```python
from build123d import *

# Parameters (mm, degrees)
SKETCH_1_R      = 1.5
EXTRUDE_1_DEPTH = 4


with BuildPart() as part:
    # 草图1 → 凸台-拉伸1 (new body)
    with BuildSketch(Plane.XY):
        with BuildLine():
            Line((46.801771952, 35.924840183), (49.578148254, 38.05597477))
            ThreePointArc((49.578148254, 38.05597477), (-61.863840118, -8.894677392), (58.29149197, -22.546661925))
            Line((58.29149197, -22.546661925), (55.027168419, -21.284048857))
            ThreePointArc((55.027168419, -21.284048857), (50.484575742, -23.055533222), (52.120542762, -27.648671255))
            ThreePointArc((52.120542762, -27.648671255), (44.589224887, -38.636783303), (34.784774262, -47.65521461))
            ThreePointArc((34.784774262, -47.65521461), (30.005565369, -46.689571072), (28.898590503, -51.438035217))
            ThreePointArc((28.898590503, -51.438035217), (16.622220854, -56.610085443), (3.498460053, -58.896186441))
            ThreePointArc((3.498460053, -58.896186441), (0, -55.5), (-3.498460053, -58.896186441))
            ThreePointArc((-3.498460053, -58.896186441), (-16.622220854, -56.610085443), (-28.898590503, -51.438035217))
            ThreePointArc((-28.898590503, -51.438035217), (-30.005565369, -46.689571072), (-34.784774262, -47.65521461))
            ThreePointArc((-34.784774262, -47.65521461), (-44.589224887, -38.636783303), (-52.120542762, -27.648671255))
            ThreePointArc((-52.120542762, -27.648671255), (-50.484575742, -23.055533222), (-55.027168419, -21.284048857))
            ThreePointArc((-55.027168419, -21.284048857), (-58.399465071, -8.396575458), (-58.794590961, 4.918950474))
            ThreePointArc((-58.794590961, 4.918950474), (-54.935090024, 7.898473524), (-57.798825407, 11.844652023))
            ThreePointArc((-57.798825407, 11.844652023), (-53.668287726, 24.509485767), (-46.801771952, 35.924840183))
            ThreePointArc((-46.801771952, 35.924840183), (-41.944101377, 36.344770734), (-42.219763715, 41.212759575))
            ThreePointArc((-42.219763715, 41.212759575), (-31.89780823, 49.633958437), (-19.949721034, 55.524846967))
            ThreePointArc((-19.949721034, 55.524846967), (-15.636156905, 53.251860036), (-13.236225354, 57.496107158))
            ThreePointArc((-13.236225354, 57.496107158), (0, 59), (13.236225354, 57.496107158))
            ThreePointArc((13.236225354, 57.496107158), (15.636156905, 53.251860036), (19.949721034, 55.524846967))
            ThreePointArc((19.949721034, 55.524846967), (31.89780823, 49.633958437), (42.219763715, 41.212759575))
            ThreePointArc((42.219763715, 41.212759575), (41.944101377, 36.344770734), (46.801771952, 35.924840183))
        make_face()
        with Locations((0, -59)):
            Circle(SKETCH_1_R, mode=Mode.SUBTRACT)
        with Locations((-31.89780823, -49.633958437)):
            Circle(SKETCH_1_R, mode=Mode.SUBTRACT)
        with Locations((-53.668287726, -24.509485767)):
            Circle(SKETCH_1_R, mode=Mode.SUBTRACT)
        with Locations((-58.399465071, 8.396575458)):
            Circle(SKETCH_1_R, mode=Mode.SUBTRACT)
        with Locations((-44.589224887, 38.636783303)):
            Circle(SKETCH_1_R, mode=Mode.SUBTRACT)
        with Locations((-16.622220854, 56.610085443)):
            Circle(SKETCH_1_R, mode=Mode.SUBTRACT)
        with Locations((16.622220854, 56.610085443)):
            Circle(SKETCH_1_R, mode=Mode.SUBTRACT)
        with Locations((44.589224887, 38.636783303)):
            Circle(SKETCH_1_R, mode=Mode.SUBTRACT)
        with Locations((53.668287726, -24.509485767)):
            Circle(SKETCH_1_R, mode=Mode.SUBTRACT)
        with Locations((31.89780823, -49.633958437)):
            Circle(SKETCH_1_R, mode=Mode.SUBTRACT)
    extrude(amount=EXTRUDE_1_DEPTH)


solid = part.part
```
Source: CAD feature listing. Evaluate the final solid. Frame: model axes, mm. A direction names the side the tool comes from. Round coordinates to 2 decimals unless told otherwise and drop trailing zeros. Loops run counter-clockwise (first coordinate to the right, second up) from the corner with the lowest first, then second, coordinate; pieces in that order, holes last.
(1) Access query for faces 1 (the cylindrical face through (-44.467, -38.778, 1.972)), 2 (the flat face through (56.682, -21.924, 1.972)). Directions: +Z, -Z, +X, -X, +Y, -Y. A direction counts if a zero-diameter tool reaches every point of the face in a straight line with its end or side. Return the directions, or none.
From the geometry:
face 1: +Z, -Z
face 2: +Z, -Z, +X, +Y
(2) Contact query for flat-ended pins moving along their axis: pin 1 Ø2.5 at (x, y) = (0, -59) entering from -Z; pin 2 Ø1.5 at (y, z) = (-20, 0.5) entering from -X; pin 3 Ø1.5 at (x, z) = (-17, 3.5) entering from -Y; pin 4 Ø2 at (y, z) = (-27.5, 3) entering from -X. Output: stop coordinate, or through.
From the geometry:
pin 1: passes through
pin 2: stops at x = -59.46
pin 3: stops at y = -60.35
pin 4: stops at x = -56.6
(3) Section query A-A (x = 0). Output: boundary loops of the cut face in (y, z).
From the geometry:
outline: (-62.5, 0) - (-60.5, 0) - (-60.5, 4) - (-62.5, 4) - close; (-57.5, 0) - (-55.5, 0) - (-55.5, 4) - (-57.5, 4) - close; (59, 0) - (62.5, 0) - (62.5, 4) - (59, 4) - close
(4) Pull-direction query (X, two-part tool) for faces 3 (the flat face through (48.2, 37, 2)), 4 (the cylindrical face through (-56.97, 8.85, 1.97)), 5 (the flat face through (-52, -23, 0)); classes: +X half, -X half, draft (parallel to the pull), parting line (faces both ways), or undercut.
From the geometry:
face 3: +X half
face 4: undercut
face 5: draft
(5) Section query D-D (z = 0.9). Give the number of separate pieces and of enclosed holes in the cut face, and give its area (3 significant figures).
From the geometry:
separate pieces: 1
enclosed holes: 10
area: 1,240 mm2
(6) Section query B-B (y = 43). Output: boundary loops of the cut face in (x, z).
From the geometry:
outline: (-45.36, 0) - (-40.4, 0) - (-40.4, 4) - (-45.36, 4) - close; (40.4, 0) - (45.36, 0) - (45.36, 4) - (40.4, 4) - close
(7) Section query C-C (x = 38.5). Output: boundary loops of the cut face in (y, z), and give its area (3 significant figures).
From the geometry:
outline: (-49.23, 0) - (-44.71, 0) - (-44.71, 4) - (-49.23, 4) - close; (44.71, 0) - (49.23, 0) - (49.23, 4) - (44.71, 4) - close
area: 36.2 mm2
(8) Material intervals for probe 1 along Y at (x, z) = (-43.5, 0.8); probe 2 along X at (y, z) = (-24, 1.65); probe 3 along Y at (x, z) = (32.5, 3.7), sorted ascending.
From the geometry:
probe 1: y = -44.88 to -39.86, 35.31 to 37.61, 39.67 to 44.88
probe 2: x = -57.71 to -55.08, -52.26 to -50.21, 50.21 to 52.26, 55.08 to 57.71
probe 3: y = -53.39 to -51.01, -48.26 to -46.19, 49.24 to 53.39
